from build123d import *

# Parameters (mm, degrees)
F0_W      = 25
F0_H      = 40
F0_R      = 6.25
F1_DEPTH  = 3.2
F2_W      = 25
F2_H      = 40
F3_DEPTH  = 40
F4_W      = 15
F4_H      = 46.4
F4_R      = 2.25
F5_DEPTH  = 5
F6_SIZE   = 2
F7_R      = 2.25
F8_DEPTH  = 3.2
F9_W      = 46.4
F9_H      = 70
F10_DEPTH = 36.8
F11_W     = 25
F11_H     = 40
F12_DEPTH = 3.2
F13_R     = 7.5
F14_DEPTH = 4


with BuildPart() as f1:
    # F0 (on Top) → F1 (new body)
    with BuildSketch(Plane.XY):
        Rectangle(F0_W, F0_H)
        Circle(F0_R, mode=Mode.SUBTRACT)
    extrude(amount=F1_DEPTH)

    # F2 (on face) → F3 (join)
    with BuildSketch(Plane.XY.offset(3.2)):
        with BuildLine():
            Line((15.7, -23.2), (15.7, 23.2))
            Line((15.7, 23.2), (7.5, 23.2))
            Line((7.5, 23.2), (7.5, 27.5))
            ThreePointArc((7.5, 27.5), (0, 35), (-7.5, 27.5))
            Line((-7.5, 27.5), (-7.5, 23.2))
            Line((-7.5, 23.2), (-15.7, 23.2))
            Line((-15.7, 23.2), (-15.7, -23.2))
            Line((-15.7, -23.2), (-7.5, -23.2))
            Line((-7.5, -23.2), (-7.5, -27.5))
            ThreePointArc((-7.5, -27.5), (0, -35), (7.5, -27.5))
            Line((7.5, -27.5), (7.5, -23.2))
            Line((7.5, -23.2), (15.7, -23.2))
        make_face()
        Polygon((-3.435234, -27.5), (-1.717617, -24.525), (1.717617, -24.525), (3.435234, -27.5), (1.717617, -30.475), (-1.717617, -30.475), align=None, mode=Mode.SUBTRACT)
        Rectangle(F2_W, F2_H, mode=Mode.SUBTRACT)
        Polygon((-3.435234, 27.5), (-1.717617, 30.475), (1.717617, 30.475), (3.435234, 27.5), (1.717617, 24.525), (-1.717617, 24.525), align=None, mode=Mode.SUBTRACT)
    extrude(amount=-F3_DEPTH)

    # F4 (on face) → F5 (join)
    with BuildSketch(Plane.XY.offset(3.2)):
        with Locations((-23.2, 0)):
            Rectangle(F4_W, F4_H)
        with Locations((-23.2, -13.2)):
            Circle(F4_R, mode=Mode.SUBTRACT)
        with Locations((-23.2, 13.2)):
            Circle(F4_R, mode=Mode.SUBTRACT)
    extrude(amount=-F5_DEPTH)

    # F6
    f6_edges = [f1.edges().sort_by_distance(p)[0] for p in [
        (15.7, 23.2, -16.8),
        (-15.7, 23.2, -19.3),
        (-15.7, -23.2, -19.3),
        (15.7, -23.2, -16.8),
        (-30.7, 23.2, 0.7),
        (-30.7, -23.2, 0.7),
    ]]
    chamfer(f6_edges, length=F6_SIZE)

    # F7 (on face) → F8 (join)
    with BuildSketch(Plane(origin=(0, 0, -36.8), x_dir=(1, 0, 0), z_dir=(0, 0, -1))):
        Polygon((1.717617, 30.475), (-1.717617, 30.475), (-3.435234, 27.5), (-1.717617, 24.525), (1.717617, 24.525), (3.435234, 27.5), align=None)
        with Locations((0, 27.5)):
            Circle(F7_R, mode=Mode.SUBTRACT)
        Polygon((-3.435234, -27.5), (-1.717617, -30.475), (1.717617, -30.475), (3.435234, -27.5), (1.717617, -24.525), (-1.717617, -24.525), align=None)
        with Locations((0, -27.5)):
            Circle(F7_R, mode=Mode.SUBTRACT)
    extrude(amount=-F8_DEPTH)

    # F9 (on face) → F10 (cut)
    with BuildSketch(Plane.XY.offset(3.2)):
        with Locations((-7.5, 0)):
            Rectangle(F9_W, F9_H)
    extrude(amount=-F10_DEPTH, mode=Mode.SUBTRACT)

    # F11 (on face) → F12 (join)
    with BuildSketch(Plane.XY.offset(-33.6)):
        Rectangle(F11_W, F11_H)
        with BuildLine():
            ThreePointArc((-6, 10), (0, 16), (6, 10))
            Line((6, 10), (6, -2.5))
            ThreePointArc((6, -2.5), (0, -8.5), (-6, -2.5))
            Line((-6, -2.5), (-6, 10))
        make_face(mode=Mode.SUBTRACT)
    extrude(amount=-F12_DEPTH)

    # F13 (on face) → F14 (join)
    with BuildSketch(Plane.XY.offset(-33.6)):
        with Locations((0, 27.5)):
            Circle(F13_R)
        Polygon((-3.435234, 27.5), (-1.717617, 30.475), (1.717617, 30.475), (3.435234, 27.5), (1.717617, 24.525), (-1.717617, 24.525), align=None, mode=Mode.SUBTRACT)
        with Locations((0, -27.5)):
            Circle(F13_R)
        Polygon((-3.435234, -27.5), (-1.717617, -24.525), (1.717617, -24.525), (3.435234, -27.5), (1.717617, -30.475), (-1.717617, -30.475), align=None, mode=Mode.SUBTRACT)
    extrude(amount=F14_DEPTH)


solid = f1.part
The model under review builds one solid part; all positions refer to its coordinate system, in mm. A direction names the side the tool comes from. Give positions to 0.01 mm unless a question says otherwise; leave off trailing zeros. Loops run counter-clockwise (first coordinate to the right, second up) from the corner with the lowest first, then second, coordinate; pieces in that order, holes last. Notation, with made-up numbers: (51.5, 15.5) -> (97.5, 15.5) arc R13 cw to (97.5, 26.5) -> close; hole circle Ø3 at (24, 17). An arc over 180 degrees is marked (long way). Put each result on its own line as item: value. Start each with the question number.
1. Clearance check with flat-ended pins moving along their axes: P1, Ø1.5, axis at x = -1.5, z = -32, coming from the +Y side; P2, Ø1, axis at x = -11.5, z = -35.5, coming from the -Y side; P3, Ø2.5, axis at x = 12, z = -36, coming from the +Y side; P4, Ø4, axis at x = 0, y = -27.5, coming from the -Z side (1 decimal). State where each tip first meets the part, or that it passes through.
2. We need section D-D on z = -36. State the section outline as (x, y) points.
3. Wall thickness on probe 1 along Y at (x, z) = (0, -35.7); probe 2 along X at (y, z) = (27.5, -34.45); probe 3 along Y at (x, z) = (-1.5, -33) (3 decimals): over which ranges is each line inside the solid? List them lowest first.
4. Mouldability with a two-part tool opening along X and no side actions: class faces 1 (the face through (7.5, -25, -35)), 2 (the face through (-0.488, -25.304, -35.222)), 3 (the face through (2, 26, -33.6)), 4 (the face through (-14.7, 22.2, -35.2)) as released by +X, released by -X, zero draft, split by the parting line, or undercut.
5. We need section B-B on y = 2.5. State the section outline as (x, z) points.
6. For faces 5 (the face through (0, 16, -35)), 6 (the face through (-7.5, -25, -35)), 7 (the face through (-2.564, 25.992, -31.628)), list the 3-axis set-ups (+Z, -Z, +X, -X, +Y, -Y) from which the entire face can be reached by the end or side of a thin tool; tool diameter is ignored.
7. We need section A-A on z = -30.25. State the section outline as (x, y) points (3 decimals), then the cut area to 3 significant figures.
8. We need section C-C on x = 0. State the section outline as (y, z) points (3 decimals).
Determined:
1. P1: y = 34.96
1. P2: y = -23.2
1. P3: y = 23.2
1. P4: through
2. outline: (-15.7, -21.2) -> (-13.7, -23.2) -> (-7.5, -23.2) -> (-7.5, -27.5) arc R7.5 ccw to (7.5, -27.5) -> (7.5, -23.2) -> (13.7, -23.2) -> (15.7, -21.2) -> (15.7, 21.2) -> (13.7, 23.2) -> (7.5, 23.2) -> (7.5, 27.5) arc R7.5 ccw to (-7.5, 27.5) -> (-7.5, 23.2) -> (-13.7, 23.2) -> (-15.7, 21.2) -> close; hole (-6, -2.5) arc R6 ccw to (6, -2.5) -> (6, 10) arc R6 ccw to (-6, 10) -> close; hole circle Ø4.5 at (0, -27.5); hole circle Ø4.5 at (0, 27.5)
3. probe 1: -35 to -29.75, -25.25 to -8.5, 16 to 25.25, 29.75 to 35
3. probe 2: -7.5 to -2.25, 2.25 to 7.5
3. probe 3: -34.848 to -30.475, -24.525 to -20.152, 20.152 to 24.525, 30.475 to 34.848
4. face 1: released by +X
4. face 2: undercut
4. face 3: undercut
4. face 4: released by -X
5. outline: (-15.7, -36.8) -> (-6, -36.8) -> (-6, -33.6) -> (-15.7, -33.6) -> close; (6, -36.8) -> (15.7, -36.8) -> (15.7, -33.6) -> (6, -33.6) -> close
6. face 5: +Z, -Z
6. face 6: +Z, -Z, -X, -Y
6. face 7: +Z
7. outline: circle Ø15 at (0, -27.5); circle Ø15 at (0, 27.5); hole (-3.435, -27.5) -> (-1.718, -30.475) -> (1.718, -30.475) -> (3.435, -27.5) -> (1.718, -24.525) -> (-1.718, -24.525) -> close; hole (-3.435, 27.5) -> (-1.718, 24.525) -> (1.718, 24.525) -> (3.435, 27.5) -> (1.718, 30.475) -> (-1.718, 30.475) -> close
7. area: 292 mm^2
8. outline: (-35, -36.8) -> (-29.75, -36.8) -> (-29.75, -33.6) -> (-30.475, -33.6) -> (-30.475, -29.6) -> (-35, -29.6) -> close; (-25.25, -36.8) -> (-8.5, -36.8) -> (-8.5, -33.6) -> (-20, -33.6) -> (-20, -29.6) -> (-24.525, -29.6) -> (-24.525, -33.6) -> (-25.25, -33.6) -> close; (16, -36.8) -> (25.25, -36.8) -> (25.25, -33.6) -> (24.525, -33.6) -> (24.525, -29.6) -> (20, -29.6) -> (20, -33.6) -> (16, -33.6) -> close; (29.75, -36.8) -> (35, -36.8) -> (35, -29.6) -> (30.475, -29.6) -> (30.475, -33.6) -> (29.75, -33.6) -> close
